Autodesk Inventor part; units mm, degrees
ref_plane "YZ Plane" through (0, 0, 0) normal (1, 0, 0) x (0, 1, 0)
ref_plane "XZ Plane" through (0, 0, 0) normal (0, 1, 0) x (-1, 0, 0)
ref_plane "XY Plane" through (0, 0, 0) normal (0, 0, 1) x (1, 0, 0)
sketch "Sketch1" plane through (0, 0, 0) normal (0, 0, 1) x (1, 0, 0)
  circle A0 centre (9.0361, 0) radius 0.5
  arc A1 (9.1111, -1.9923) -> (9.1111, 1.9923) centre (8.9361, 0) ccw
  circle A2 centre (8.9361, 0) radius 2
  point P0 (0, 0)
  point P1 (9.1111, 1.9923)
  point P2 (9.1111, -1.9923)
extrude "Extrusion1" add sketch "Sketch1" along normal blind 4
sketch "Sketch2" plane through (8.9361, 0, 0) normal (0, 0, -1) x (-1, 0, 0)
  circle A0 centre (0, 0) radius 2
  circle A1 centre (-0.1, 0) radius 0.5
  point P0 (8.9361, 0)
extrude "Extrusion2" cut sketch "Sketch2" against normal blind 0.5
sketch "Sketch3" plane through (8.9361, 0, 0.5) normal (0, 0, -1) x (-1, 0, 0)
  circle A0 centre (34.6774, 22.9773) radius 1.5
  arc A1 (36.9746, 24.9067) -> (34.2673, 20.0054) centre (34.6774, 22.9773) ccw
  circle A2 centre (34.6774, 22.9773) radius 3
  circle A3 centre (41.0489, 27.7862) radius 1.5
  circle A4 centre (41.0489, 27.7862) radius 3
  point P0 (8.9361, 0)
  point P1 (34.2673, 20.0054)
  dimension "d11" = 3
  dimension "d12" = 6
extrude "Extrusion3" add sketch "Sketch3" against normal up to surface (3.5 mm away) contours A4
sketch "Sketch6" plane through (8.9361, 0, 0.5) normal (0, 0, -1) x (-1, 0, 0)
  circle A0 centre (41.0489, 27.7862) radius 3
  circle A1 centre (41.0489, 27.7862) radius 1.5
  circle A2 centre (0, 0) radius 2
  circle A3 centre (-0.1, 0) radius 0.5
  line L0 (-1.1543, 1.6333) -> (39.3175, 30.2361)
  line L1 (1.0875, -1.6785) -> (42.6801, 25.2684)
  point P0 (8.9361, 0)
extrude "Extrusion6" add sketch "Sketch6" against normal blind 1.75 contours A0 L1 A2 L0
sketch "Sketch7" plane through (8.9361, 0, 2.25) normal (0, 0, 1) x (1, 0, 0)
  line L0 (1.1543, 1.6333) -> (-39.3175, 30.2361)
  circle A0 centre (-41.0489, 27.7862) radius 3
  circle A1 centre (0, 0) radius 2
  circle A2 centre (0.1, 0) radius 0.5
  line L1 (0.1, 0) -> (-41.0489, 27.7862)
  point P0 (-8.9361, 0)
  point P1 (-38.5627, 26.1073)
  point P2 (-1.6255, 1.1652)
extrude "Extrusion7" add sketch "Sketch7" along normal up to surface (1.75 mm away) contours A1 L1 A0 L0
properties part number "ServoShaft_3DPrint"
Geometry: final body of the model. Coordinates: model frame, mm. Give positions to 0.01 mm unless a question says otherwise; leave off trailing zeros. Loops run counter-clockwise (first coordinate to the right, second up) from the corner with the lowest first, then second, coordinate; pieces in that order, holes last. Notation, with made-up numbers: (11.25, -34) - (69.25, -34) arc R19 cw to (69.25, -18) - close; hole circle Ø3 at (-8, -0.5). An arc over 180 degrees is marked (long way). Answer as CSV lines item,"result". Start each with the question number.
(1) Section query D-D (y = 19.5). Output: boundary loops of the cut face in (x, z), and give its area (3 significant figures).
(2) Section query C-C (x = -15). Output: boundary loops of the cut face in (y, z), and give its area (3 significant figures).
(3) Section query B-B (y = 0). Output: boundary loops of the cut face in (x, z).
(4) Ray query, line 1 along Z through (x, y) = (-8.5, 11); line 2 along Y through (x, z) = (-23.5, 2.3); line 3 along X through (y, z) = (25, 1.85). Return the intervals inside material, ascending. Write a range as [from, to].
(5) Mould query, pull axis Y, two halves, no side actions, for faces 1 (the face through (7.525, -1.417, 2.614)), 2 (the face through (-12.66, 11.61, 1.36)), 3 (the face through (-12, 14, 0.5)). Classes: +Y half, -Y half, draft (parallel to the pull), parting line (faces both ways), or undercut.
(6) Pin query (flat end, axial travel): P1, Ø5, axis at x = -13.5, y = 12, coming from the +Z side; P2, Ø1.5, axis at x = -7, z = 1.5, coming from the -Y side; P3, Ø1.5, axis at y = 17, z = 2, coming from the +X side. Return the tip coordinate at first contact, or that it passes through.
(7) Section query A-A (z = 1.45). Output: boundary loops of the cut face in (x, y), and give its area (3 significant figures).
Worked answers:
1,outline,"(-24.84, 0.5) - (-15.19, 0.5) - (-15.19, 4) - (-19.84, 4) - (-19.84, 2.25) - (-24.84, 2.25) - close"
1,area,"25.0 mm^2"
2,outline,"(13.12, 0.5) - (19.37, 0.5) - (19.37, 4) - (16.23, 4) - (16.23, 2.25) - (13.12, 2.25) - close"
2,area,"16.4 mm^2"
3,outline,"(5.26, 0.5) - (8.54, 0.5) - (8.54, 4) - (6.94, 4) - (6.94, 2.25) - (5.26, 2.25) - close; (9.54, 0.5) - (10.94, 0.5) - (10.94, 4) - (9.54, 4) - close"
4,line 1,"z = [0.5, 2.25]"
4,line 2,"y = [21.97, 25.37]"
4,line 3,"x = [-33.33, -22.97]"
5,face 1,"undercut"
5,face 2,"-Y half"
5,face 3,"draft"
6,P1,"stops at z = 2.25"
6,P2,"stops at y = 7.46"
6,P3,"stops at x = -10.59"
7,outline,"(-33.74, 25.27) - (7.85, -1.68) arc R2 ccw to (9.11, -1.99) arc R2 ccw to (10.09, 1.63) - (-30.38, 30.24) arc R3 ccw (long way) to start; hole circle Ø3 at (-32.11, 27.79); hole circle Ø1 at (9.04, 0)"
7,area,"260 mm^2"
